Geometry: final body of the model. Coordinates: model frame, mm. A direction names the side the tool comes from. Round coordinates to 2 decimals unless told otherwise and drop trailing zeros. Order: outer loops, then holes, each group sorted by start corner. A loop starts at its lowest first (then second) coordinate and runs counter-clockwise, first axis right, second up. Notation, with made-up numbers: (17.25, -3.5) -> (60.25, -3.5) arc R23 ccw to (60.25, 35.5) -> close; hole circle Ø6 at (-19.5, 83). An arc over 180 degrees is marked (long way). Put each result on its own line as item: value.
```python
from build123d import *

# Parameters (mm, degrees)
BOSS_EXTRUDE1_START = -40
SKETCH2_W           = 59.507
SKETCH2_H           = 48.644
BOSS_EXTRUDE1_DEPTH = 20
SKETCH3_W           = 63.507
SKETCH3_H           = 52.644
BOSS_EXTRUDE2_DEPTH = 2
SKETCH12_W          = 5
SKETCH12_H          = 5
SKETCH12_W_2        = 6
SKETCH12_H_2        = 5.5
BOSS_EXTRUDE4_DEPTH = 6
SKETCH20_R          = 1.1
CUT_EXTRUDE12_DEPTH = 10
SKETCH23_W          = 5
SKETCH23_H          = 48.644
CUT_EXTRUDE13_DEPTH = 5
SKETCH25_R          = 1.25
CUT_EXTRUDE14_DEPTH = 73
SKETCH27_W          = 4.650000165
SKETCH27_H          = 8.443476487
CUT_EXTRUDE15_DEPTH = 3
SKETCH28_W          = 3.45
SKETCH28_H          = 9.6
SKETCH28_W_2        = 3.86148
SKETCH28_H_2        = 9.589284943
CUT_EXTRUDE16_DEPTH = 3
SKETCH30_R          = 1.25
CUT_EXTRUDE24_DEPTH = 3
FILLET1_R           = 1
FILLET2_R           = 1
FILLET3_R           = 1
FILLET4_R           = 1


with BuildPart() as part:
    # Sketch2 → Boss-Extrude1 (new body)
    with BuildSketch(Plane.XY.offset(BOSS_EXTRUDE1_START)):
        Polygon((60.436010502, 80.424), (121.572, 80.424), (121.572, 27.78), (58.065, 27.78), (58.065, 80.424), align=None)
        with Locations((89.8185, 54.102)):
            Rectangle(SKETCH2_W, SKETCH2_H, mode=Mode.SUBTRACT)
    extrude(amount=BOSS_EXTRUDE1_DEPTH)

    # Sketch3 → Boss-Extrude2 (add)
    with BuildSketch(Plane(origin=(0, 0, -40), x_dir=(-1, 0, 0), z_dir=(0, 0, -1))):
        with Locations((-89.8185, 54.102)):
            Rectangle(SKETCH3_W, SKETCH3_H)
    extrude(amount=BOSS_EXTRUDE2_DEPTH)

    # Sketch12 → Boss-Extrude4 (add)
    with BuildSketch(Plane.XY.offset(-40)):
        with Locations((62.565, 75.924)):
            Rectangle(SKETCH12_W, SKETCH12_H)
        with Locations((116.572, 75.924)):
            Rectangle(SKETCH12_W_2, SKETCH12_H)
        with Locations((117.072, 32.53)):
            Rectangle(SKETCH12_W, SKETCH12_H_2)
        with Locations((62.565, 32.28)):
            Rectangle(SKETCH12_W, SKETCH12_H)
    extrude(amount=BOSS_EXTRUDE4_DEPTH)

    # Sketch20 → Cut-Extrude12 (cut)
    with BuildSketch(Plane.XY.offset(-34)):
        with Locations((62.836, 75.44)):
            Circle(SKETCH20_R)
        with Locations((115.905, 75.538)):
            Circle(SKETCH20_R)
        with Locations((117.094, 33.147)):
            Circle(SKETCH20_R)
        with Locations((62.455, 32.641)):
            Circle(SKETCH20_R)
    extrude(amount=-CUT_EXTRUDE12_DEPTH, mode=Mode.SUBTRACT)

    # Sketch23 → Cut-Extrude13 (cut)
    with BuildSketch(Plane(origin=(60.065, 0, 0), x_dir=(0, 0, -1), z_dir=(1, 0, 0))):
        with Locations((22.5, 54.102)):
            Rectangle(SKETCH23_W, SKETCH23_H)
    extrude(amount=-CUT_EXTRUDE13_DEPTH, mode=Mode.SUBTRACT)

    # Sketch25 → Cut-Extrude14 (cut)
    with BuildSketch(Plane(origin=(0, 80.424, 0), x_dir=(1, 0, 0), z_dir=(0, 1, 0))):
        with Locations(Location((60.565, 21.7, 0), (0, 0, 270))):
            Circle(SKETCH25_R)
    extrude(amount=-CUT_EXTRUDE14_DEPTH, mode=Mode.SUBTRACT)

    # Sketch27 → Cut-Extrude15 (cut)
    with BuildSketch(Plane(origin=(121.572, 0, 0), x_dir=(0, 0, -1), z_dir=(1, 0, 0))):
        with Locations((36.324999988, 44.82384952)):
            Rectangle(SKETCH27_W, SKETCH27_H)
    extrude(amount=-CUT_EXTRUDE15_DEPTH, mode=Mode.SUBTRACT)

    # Sketch28 → Cut-Extrude16 (cut)
    with BuildSketch(Plane.ZY.offset(-58.065)):
        with Locations((-35.725, 51.339048194)):
            Rectangle(SKETCH28_W, SKETCH28_H)
        with Locations((-35.51926, 39.648781472)):
            Rectangle(SKETCH28_W_2, SKETCH28_H_2)
    extrude(amount=-CUT_EXTRUDE16_DEPTH, mode=Mode.SUBTRACT)

    # Sketch30 → Cut-Extrude24 (cut)
    with BuildSketch(Plane(origin=(119.572, 0, 0), x_dir=(0, 0, -1), z_dir=(1, 0, 0))):
        with Locations(Location((21.90078297, 52.638173314, 0), (0, 0, 180))):
            Circle(SKETCH30_R)
    extrude(amount=CUT_EXTRUDE24_DEPTH, mode=Mode.SUBTRACT)

    # Fillet1
    fillet1_edges = [part.edges().sort_by_distance(p)[0] for p in [
        (58.065, 80.424, -31),
    ]]
    fillet(fillet1_edges, radius=FILLET1_R)

    # Fillet2
    fillet2_edges = [part.edges().sort_by_distance(p)[0] for p in [
        (121.572, 80.424, -31),
    ]]
    fillet(fillet2_edges, radius=FILLET2_R)

    # Fillet3
    fillet3_edges = [part.edges().sort_by_distance(p)[0] for p in [
        (121.572, 27.78, -31),
    ]]
    fillet(fillet3_edges, radius=FILLET3_R)

    # Fillet4
    fillet4_edges = [part.edges().sort_by_distance(p)[0] for p in [
        (58.065, 27.78, -31),
    ]]
    fillet(fillet4_edges, radius=FILLET4_R)


solid = part.part
```
1. Cut plane D-D on y = 69. Return loops of the section in (x, z) (3 decimals), and give its area (3 significant figures).
Ans:
outline: (58.065, -42) -> (121.572, -42) -> (121.572, -20) -> (119.572, -20) -> (119.572, -40) -> (60.065, -40) -> (60.065, -25) -> (58.065, -25) -> close
area: 197 mm²
2. Contact query for flat-ended pins moving along their axis: P1, Ø1.5, axis at y = 48, z = -37.5, coming from the +X side (3 decimals); P2, Ø1.3, axis at x = 117.094, y = 33.147, coming from the -Z side; P3, Ø4, axis at x = 115, y = 75, coming from the +Z side; P4, Ø10, axis at x = 98.5, y = 72.5, coming from the +Z side. Output: stop coordinate, or through.
Ans:
P1: x = 60.065
P2: through
P3: z = -34
P4: z = -40
3. Cut plane A-A on y = 37. Return loops of the section in (x, z) (3 decimals), and give its area (3 significant figures).
Ans:
outline: (58.065, -42) -> (121.572, -42) -> (121.572, -20) -> (119.572, -20) -> (119.572, -40) -> (60.065, -40) -> (60.065, -37.45) -> (58.065, -37.45) -> close; (58.065, -33.589) -> (60.065, -33.589) -> (60.065, -25) -> (58.065, -25) -> close
area: 189 mm²
4. Material intervals for probe 1 along X at (y, z) = (75.44, -39) (3 decimals); probe 2 along Y at (x, z) = (98, -21.75); probe 3 along X at (y, z) = (46.5, -27.5) (3 decimals), sorted ascending.
Ans:
probe 1: 58.065 to 61.736, 63.936 to 65.065, 113.572 to 114.809, 117.001 to 121.572
probe 2: 27.78 to 29.78, 78.42 to 80.42
probe 3: 58.065 to 60.065, 119.572 to 121.572
5. Cut plane B-B on x = 84. Return loops of the section in (y, z).
Ans:
outline: (27.78, -42) -> (80.42, -42) -> (80.42, -20) -> (78.42, -20) -> (78.42, -40) -> (29.78, -40) -> (29.78, -20) -> (27.78, -20) -> close
6. Draft query along Z for faces 4 (the face through (59, 34.854, -36)), 5 (the face through (63.852, 75.019, -37.944)), 6 (the face through (63, 77, -34)). Return one class per face: +Z half, -Z half, draft (parallel to the pull), parting line (faces both ways), or undercut.
Ans:
face 4: undercut
face 5: draft
face 6: +Z half
7. Cut plane C-C on z = -21.7. Return loops of the section in (x, y) (3 decimals).
Ans:
outline: (58.065, 28.78) arc R1 ccw to (59.065, 27.78) -> (59.315, 27.78) -> (59.315, 29.78) -> (58.065, 29.78) -> close; (58.065, 78.424) -> (59.315, 78.424) -> (59.315, 80.424) -> (59.065, 80.424) arc R1 ccw to (58.065, 79.424) -> close; (61.815, 27.78) -> (120.572, 27.78) arc R1 ccw to (121.572, 28.78) -> (121.572, 51.404) -> (119.572, 51.404) -> (119.572, 29.78) -> (61.815, 29.78) -> close; (61.815, 78.424) -> (119.572, 78.424) -> (119.572, 53.872) -> (121.572, 53.872) -> (121.572, 79.424) arc R1 ccw to (120.572, 80.424) -> (61.815, 80.424) -> close
8. Set-up query: faces 1 (the face through (121, 40.602, -36)), 2 (the face through (117, 35.28, -37)), 3 (the face through (59, 46.539, -36)). Return all of +Z, -Z, +X, -X, +Y, -Y with unobstructed straight access to the full face (end or side cutting, diameter ignored); none if empty.
Ans:
face 1: +X
face 2: +Z
face 3: +X, -X
